Check sheet for the modelled part. Datum: model origin and axes. Units: mm. Face numbers are marked on the shaded views. A direction names the side the tool comes from. Round coordinates to 2 decimals unless told otherwise and drop trailing zeros. Write each loop counter-clockwise with the first axis right and the second up, starting at its lowest first coordinate (ties: lowest second). Pieces come first, ordered by that corner, then holes.
Item 1: Go/stop test with flat-tipped pins: pin 1 Ø7.5 at (y, z) = (19.5, -17.5) entering from -X; pin 2 Ø10 at (x, z) = (-2, -30) entering from +Y; pin 3 Ø2 at (x, y) = (-10.5, 19.5) entering from +Z. Record where each tip stops, or that it passes through.
Item 2: Cross-section at C-C on y = 21. Enter the section's corners in (x, z), plus the area to 3 significant figures.
Item 3: Release check for a two-part mould opening along X. For the marked faces 3, 4, 5 and 6 record: +X half, -X half, draft (parallel to the pull), parting line (faces both ways), or undercut.
Item 4: Cross-section at D-D on y = 3.5. Enter the section's corners in (x, z).
Item 5: Cross-section at A-A on z = -6. Enter the section's corners in (x, y).
Item 6: Tool access check on the marked faces 1 and 2. Record the directions out of +Z, -Z, +X, -X, +Y, -Y that give a thin tool (end or side, any length) a straight path to the whole face; none if there is none.
Item 7: Material ranges on line 1 (Z direction, x = -14, y = 2); line 2 (Y direction, x = -29, z = -9.5); line 3 (X direction, y = 2, z = -22), recorded low to high.
Item 8: Cross-section at B-B on x = 8.5. Enter the section's corners in (y, z).
from build123d import *

# Parameters (mm, degrees)
SKETCH_1_W          = 43
SKETCH_1_H          = 43
SKETCH_1_R          = 1.75
SKETCH_1_R_2        = 12.5
EXTRUDE_1_DEPTH     = 5
SKETCH_3_W          = 43
SKETCH_3_H          = 5
EXTRUDE_2_DEPTH     = 5
SKETCH_4_W          = 43
SKETCH_4_H          = 30
EXTRUDE_3_DEPTH     = 5
SKETCH_5_R          = 1.55
CUT_EXTRUDE_1_DEPTH = 68.028261499
EXTRUDE_4_DEPTH     = 5
SKETCH_7_W          = 20
SKETCH_7_H          = 5
CUT_EXTRUDE_2_DEPTH = 10


with BuildPart() as part:
    # 草图1 → 凸台-拉伸1 (new body)
    with BuildSketch(Plane(origin=(0, 0, 0), x_dir=(1, 0, 0), z_dir=(0, 1, 0))):
        with Locations((-14.399691358, 11.712191358)):
            Rectangle(SKETCH_1_W, SKETCH_1_H)
        with Locations(Location((1.100308642, 27.212191358, 0), (0, 0, 270))):
            Circle(SKETCH_1_R, mode=Mode.SUBTRACT)
        with Locations(Location((-29.899691358, 27.212191358, 0), (0, 0, 270))):
            Circle(SKETCH_1_R, mode=Mode.SUBTRACT)
        with Locations(Location((-29.899691358, -3.787808642, 0), (0, 0, 270))):
            Circle(SKETCH_1_R, mode=Mode.SUBTRACT)
        with Locations(Location((1.100308642, -3.787808642, 0), (0, 0, 270))):
            Circle(SKETCH_1_R, mode=Mode.SUBTRACT)
        with Locations(Location((-14.399691358, 11.712191358, 0), (0, 0, 270))):
            Circle(SKETCH_1_R_2, mode=Mode.SUBTRACT)
    extrude(amount=EXTRUDE_1_DEPTH)

    # 草图3 → 凸台-拉伸2 (add)
    with BuildSketch(Plane(origin=(0, 0, -33.212191358), x_dir=(-1, 0, 0), z_dir=(0, 0, -1))):
        with Locations((14.399691358, 2.5)):
            Rectangle(SKETCH_3_W, SKETCH_3_H)
    extrude(amount=EXTRUDE_2_DEPTH)

    # 草图4 → 凸台-拉伸3 (add)
    with BuildSketch(Plane(origin=(0, 0, -38.212191358), x_dir=(-1, 0, 0), z_dir=(0, 0, -1))):
        with Locations((14.399691358, 15)):
            Rectangle(SKETCH_4_W, SKETCH_4_H)
    extrude(amount=EXTRUDE_3_DEPTH)

    # 草图5 → 切除-拉伸1 (cut, through all)
    with BuildSketch(Plane.XY.offset(-38.212191358)):
        with Locations((-0.899691358, 10)):
            Circle(SKETCH_5_R)
        with Locations((-25.899691358, 10)):
            Circle(SKETCH_5_R)
    extrude(amount=-CUT_EXTRUDE_1_DEPTH, mode=Mode.SUBTRACT)

    # 草图6 → 凸台-拉伸4 (add)
    with BuildSketch(Plane(origin=(7.100308642, 0, 0), x_dir=(0, 0, -1), z_dir=(1, 0, 0))):
        Polygon((-9.787808642, 0), (-9.787808642, 5), (38.212191358, 30), (43.212191358, 30), (43.212191358, 0), align=None)
    extrude(amount=EXTRUDE_4_DEPTH)

    # 草图7 → 切除-拉伸2 (cut)
    with BuildSketch(Plane(origin=(0, 30, 0), x_dir=(1, 0, 0), z_dir=(0, 1, 0))):
        with Locations((-14.699691358, 40.712191358)):
            Rectangle(SKETCH_7_W, SKETCH_7_H)
    extrude(amount=-CUT_EXTRUDE_2_DEPTH, mode=Mode.SUBTRACT)


solid = part.part
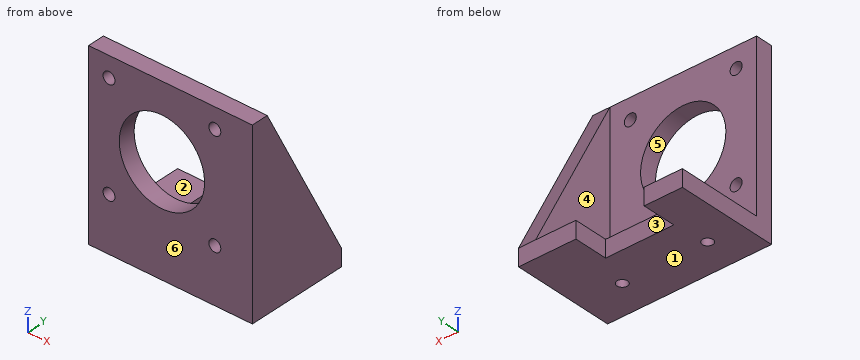
Response values:
1. pin 1: stops at x = 7.1
1. pin 2: stops at y = 5
1. pin 3: stops at z = -38.21
2. outline: (-35.9, -43.21) - (-24.7, -43.21) - (-24.7, -38.21) - (-35.9, -38.21) - close; (-4.7, -43.21) - (12.1, -43.21) - (12.1, -20.93) - (7.1, -20.93) - (7.1, -38.21) - (-4.7, -38.21) - close
2. area: 226 mm2
3. face 3: undercut
3. face 4: -X half
3. face 5: undercut
3. face 6: draft
4. outline: (-35.9, -43.21) - (12.1, -43.21) - (12.1, 9.79) - (-35.9, 9.79) - close; hole circle Ø3.5 at (-29.9, -27.21); hole circle Ø3.5 at (-29.9, 3.79); hole circle Ø25 at (-14.4, -11.71); hole circle Ø3.5 at (1.1, -27.21); hole circle Ø3.5 at (1.1, 3.79)
5. outline: (-35.9, 0) - (-25.52, 0) - (-25.52, 5) - (-35.9, 5) - close; (-3.28, 0) - (12.1, 0) - (12.1, 13.22) - (7.1, 13.22) - (7.1, 5) - (-3.28, 5) - close
6. face 1: -Z, +X, -X, +Y, -Y
6. face 2: +Z, -X, +Y
7. line 1: z = -43.21 to -24.21, 0.78 to 9.79
7. line 2: y = 0 to 5
7. line 3: x = -35.9 to -21.5, -7.3 to 12.1
8. outline: (0, -43.21) - (30, -43.21) - (30, -38.21) - (5, 9.79) - (0, 9.79) - close
